Design review of the part shown in the three views and the two pictorial views. Dimensions are in mm from the part's minimum x, y and z. A direction names the side the tool comes from. Round coordinates to 2 decimals unless told otherwise and drop trailing zeros. Write each loop counter-clockwise with the first axis right and the second up, starting at its lowest first coordinate (ties: lowest second). Pieces come first, ordered by that corner, then holes. Notation, with made-up numbers: (3, -32) - (19, -32) arc R20 cw to (19, -12) - close; hole circle Ø10 at (-22, -36.5). An arc over 180 degrees is marked (long way). One line per item, written item: value. Start each with the question number.
Q1. Add section B-B on x = 35. Write out the cut boundary in (y, z).
Q2. Add section D-D on x = 6. Write out the cut boundary in (y, z), and give its area (3 significant figures).
Q3. Mouldability with a two-part tool opening along X and no side actions: class the marked faces 4, 5 and 6 as +X half, -X half, draft (parallel to the pull), parting line (faces both ways), or undercut.
Q4. Tool access review of the marked faces 1, 2 and 3: name each direction out of +Z, -Z, +X, -X, +Y, -Y from which nothing blocks a thin tool from reaching the whole face with its end or side.
Q5. Clearance check with flat-ended pins moving along their axes: pin 1 Ø1.6 at (x, y) = (5.5, 34) entering from +Z; pin 2 Ø5 at (x, y) = (12, 12) entering from +Z; pin 3 Ø0.6 at (x, z) = (27, 5) entering from +Y; pin 4 Ø1 at (x, y) = (6.5, 25.5) entering from -Z. State where each tip first meets the part, or that it passes through.
Q6. For probe 1 along Y at (x, z) = (35, 3.25); probe 2 along X at (y, z) = (37, 2.9) (1 decimal); probe 3 along Z at (x, y) = (17, 14), list the stretches that pass through material, from the lowest coordinate up.
Q7. Add section A-A on z = 3. Give the number of separate pieces and of enclosed holes in the cut face, and give its area (3 significant figures).
Q8. Add section C-C on y = 22. Write out the cut boundary in (x, z), and give its area (3 significant figures).
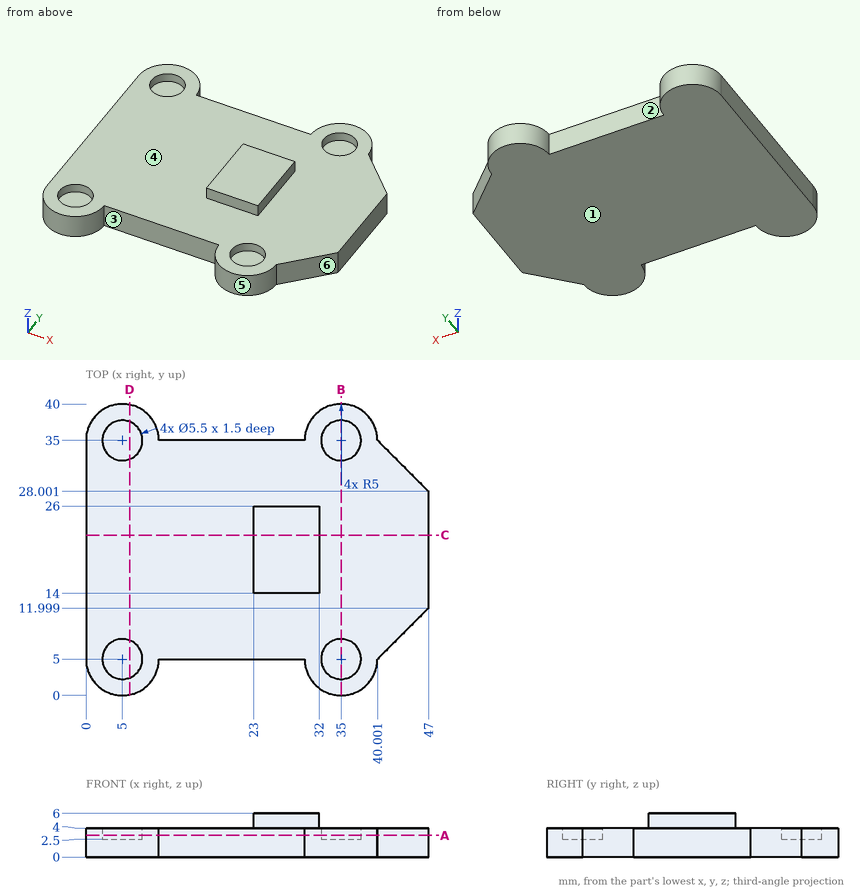
Result set:
1. outline: (0, 0) - (40, 0) - (40, 4) - (37.75, 4) - (37.75, 2.5) - (32.25, 2.5) - (32.25, 4) - (7.75, 4) - (7.75, 2.5) - (2.25, 2.5) - (2.25, 4) - (0, 4) - close
2. outline: (0.1, 0) - (39.9, 0) - (39.9, 4) - (37.56, 4) - (37.56, 2.5) - (32.44, 2.5) - (32.44, 4) - (7.56, 4) - (7.56, 2.5) - (2.44, 2.5) - (2.44, 4) - (0.1, 4) - close
2. area: 144 mm^2
3. face 4: draft
3. face 5: undercut
3. face 6: +X half
4. face 1: -Z, +X, -X, +Y, -Y
4. face 2: +Z, -Z, +Y
4. face 3: +Z, -Z, -Y
5. pin 1: stops at z = 2.5
5. pin 2: stops at z = 4
5. pin 3: stops at y = 26
5. pin 4: stops at z = 0
6. probe 1: y = 0 to 2.25, 7.75 to 32.25, 37.75 to 40
6. probe 2: x = 0.4 to 3.1, 6.9 to 9.6, 30.4 to 33.1, 36.9 to 39.6
6. probe 3: z = 0 to 4
7. separate pieces: 1
7. enclosed holes: 4
7. area: 1,420 mm^2
8. outline: (0, 0) - (47, 0) - (47, 4) - (32, 4) - (32, 6) - (23, 6) - (23, 4) - (0, 4) - close
8. area: 206 mm^2
